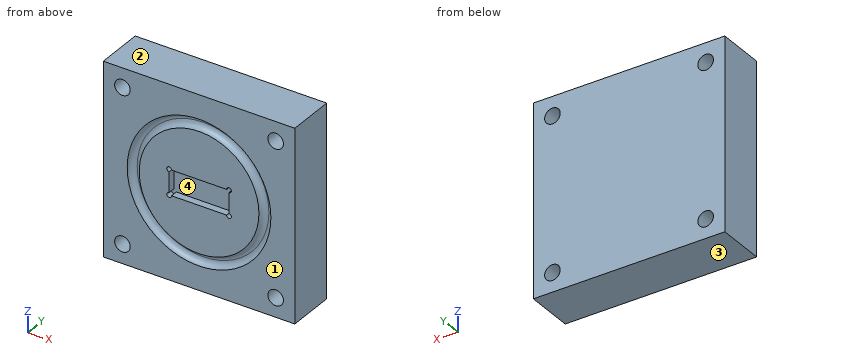
```python
from build123d import *

# Parameters (mm, degrees)
F1_W     = 80
F1_H     = 80
F2_DEPTH = 20
F4_R     = 3.25
F5_DEPTH = 20.001
F4_R_2   = 30
F4_R_3   = 25
F6_DEPTH = 2.5
F7_DEPTH = 3
F8_R     = 2.49999
F9_R     = 2.49999


# Not quite as in the source:
# - a fillet or chamfer is up to 0.001 mm smaller than in the source, because OpenCascade refuses the exact size


with BuildPart() as f2:
    # F1 (on Front) → F2 (new body)
    with BuildSketch(Plane.XZ):
        with Locations((40, 40)):
            Rectangle(F1_W, F1_H)
    extrude(amount=F2_DEPTH)

    # F4 (on face) → F5 (cut, through all)
    with BuildSketch(Plane.XZ.offset(20)):
        with Locations((72, 8)):
            Circle(F4_R)
        with Locations((8, 8)):
            Circle(F4_R)
        with Locations((8, 72)):
            Circle(F4_R)
        with Locations((72, 72)):
            Circle(F4_R)
    extrude(amount=-F5_DEPTH, mode=Mode.SUBTRACT)

    # F4 (on face) → F6 (cut)
    with BuildSketch(Plane.XZ.offset(20)):
        with Locations((40, 40)):
            Circle(F4_R_2)
        with Locations((40, 40)):
            Circle(F4_R_3, mode=Mode.SUBTRACT)
    extrude(amount=-F6_DEPTH, mode=Mode.SUBTRACT)

    # F4 (on face) → F7 (cut)
    with BuildSketch(Plane.XZ.offset(20)):
        with BuildLine():
            Line((28.5, 45.25), (27.5, 45.25))
            Line((27.5, 45.25), (27.5, 44.25))
            ThreePointArc((27.5, 44.25), (28.2071067812, 44.5428932188), (28.5, 45.25))
        make_face()
        with BuildLine():
            Line((51.5, 45.25), (28.5, 45.25))
            ThreePointArc((28.5, 45.25), (28.2071067812, 44.5428932188), (27.5, 44.25))
            Line((27.5, 44.25), (27.5, 40))
            Line((27.5, 40), (52.5, 40))
            Line((52.5, 40), (52.5, 44.25))
            ThreePointArc((52.5, 44.25), (51.7928932188, 44.5428932188), (51.5, 45.25))
        make_face()
        with BuildLine():
            Line((52.5, 45.25), (51.5, 45.25))
            ThreePointArc((51.5, 45.25), (51.7928932188, 44.5428932188), (52.5, 44.25))
            Line((52.5, 44.25), (52.5, 45.25))
        make_face()
        with BuildLine():
            ThreePointArc((28.5, 34.75), (28.2071067812, 35.4571067812), (27.5, 35.75))
            Line((27.5, 35.75), (27.5, 34.75))
            Line((27.5, 34.75), (28.5, 34.75))
        make_face()
        with BuildLine():
            Line((52.5, 40), (27.5, 40))
            Line((27.5, 40), (27.5, 35.75))
            ThreePointArc((27.5, 35.75), (28.2071067812, 35.4571067812), (28.5, 34.75))
            Line((28.5, 34.75), (51.5, 34.75))
            ThreePointArc((51.5, 34.75), (51.7928932188, 35.4571067812), (52.5, 35.75))
            Line((52.5, 35.75), (52.5, 40))
        make_face()
        with BuildLine():
            Line((52.5, 34.75), (52.5, 35.75))
            ThreePointArc((52.5, 35.75), (51.7928932188, 35.4571067812), (51.5, 34.75))
            Line((51.5, 34.75), (52.5, 34.75))
        make_face()
        with BuildLine():
            Line((27.5, 34.75), (27.5, 35.75))
            ThreePointArc((27.5, 35.75), (26.7928932188, 34.0428932188), (28.5, 34.75))
            Line((28.5, 34.75), (27.5, 34.75))
        make_face()
        with BuildLine():
            ThreePointArc((53.5, 34.75), (53.2071067812, 35.4571067812), (52.5, 35.75))
            Line((52.5, 35.75), (52.5, 34.75))
            Line((52.5, 34.75), (51.5, 34.75))
            ThreePointArc((51.5, 34.75), (52.5, 33.75), (53.5, 34.75))
        make_face()
        with BuildLine():
            ThreePointArc((53.5, 45.25), (52.5, 46.25), (51.5, 45.25))
            Line((51.5, 45.25), (52.5, 45.25))
            Line((52.5, 45.25), (52.5, 44.25))
            ThreePointArc((52.5, 44.25), (53.2071067812, 44.5428932188), (53.5, 45.25))
        make_face()
        with BuildLine():
            Line((27.5, 44.25), (27.5, 45.25))
            Line((27.5, 45.25), (28.5, 45.25))
            ThreePointArc((28.5, 45.25), (26.7928932188, 45.9571067812), (27.5, 44.25))
        make_face()
    extrude(amount=-F7_DEPTH, mode=Mode.SUBTRACT)

    # F8 (radius 2.5 in the source; OpenCascade refuses exactly that, so slightly less here)
    f8_edges = [f2.edges().sort_by_distance(p)[0] for p in [
        (15, -17.5, 40),
    ]]
    fillet(f8_edges, radius=F8_R)

    # F9 (radius 2.5 in the source; OpenCascade refuses exactly that, so slightly less here)
    f9_edges = [f2.edges().sort_by_distance(p)[0] for p in [
        (10, -17.5, 40),
    ]]
    fillet(f9_edges, radius=F9_R)


solid = f2.part
```
Source: CAD feature listing. Evaluate the final solid. Frame: model axes, mm. Face numbers are marked on the shaded views. Round coordinates to 2 decimals unless told otherwise and drop trailing zeros. Loops run counter-clockwise (first coordinate to the right, second up) from the corner with the lowest first, then second, coordinate; pieces in that order, holes last.
1. Contact query for flat-ended pins moving along their axis: pin 1 (6.5 mm diameter, centred on x = 34, z = 39, fed in from -Y); pin 2 (5 mm diameter, centred on x = 72, z = 8, fed in from +Y). Output: stop coordinate, or through.
2. Ray query, L1, parallel to Z at x = 8, y = -6.75; L2, parallel to X at y = -4, z = 75; L3, parallel to X at y = -13, z = 71. Return the intervals inside material, ascending.
3. Mould query, pull axis Z, two halves, no side actions, for the marked faces 1, 2, 3 and 4. Classes: released by +Z, released by -Z, zero draft, split by the parting line, or undercut.
4. Section query B-B on y = -3.5. Output: boundary loops of the cut face in (x, z), and give its area (3 significant figures).
5. Section query A-A on x = 72. Output: boundary loops of the cut face in (y, z), and give its area (3 significant figures).
Answers below:
1. pin 1: stops at y = -17
1. pin 2: passes through
2. L1: z = 0 to 4.75, 11.25 to 68.75, 75.25 to 80
2. L2: x = 0 to 6.75, 9.25 to 70.75, 73.25 to 80
2. L3: x = 0 to 4.91, 11.09 to 68.91, 75.09 to 80
3. face 1: zero draft
3. face 2: released by +Z
3. face 3: released by -Z
3. face 4: undercut
4. outline: (0, 0) - (80, 0) - (80, 80) - (0, 80) - close; hole circle Ø6.5 at (8, 8); hole circle Ø6.5 at (8, 72); hole circle Ø6.5 at (72, 8); hole circle Ø6.5 at (72, 72)
4. area: 6,270 mm2
5. outline: (-20, 0) - (0, 0) - (0, 4.75) - (-20, 4.75) - close; (-20, 11.25) - (0, 11.25) - (0, 68.75) - (-20, 68.75) - close; (-20, 75.25) - (0, 75.25) - (0, 80) - (-20, 80) - close
5. area: 1,340 mm2
